Read the model definition and answer for the solid it produces. Units are mm, in the model's axes. Give positions to 0.01 mm unless a question says otherwise; leave off trailing zeros. Write each loop counter-clockwise with the first axis right and the second up, starting at its lowest first coordinate (ties: lowest second). Pieces come first, ordered by that corner, then holes. Notation, with made-up numbers: M 84.25,26.5 L 111.25,26.5 A6 cw 111.25,33.5 Z; hole C -11,8 d1. An arc over 180 degrees is marked long. Use a Markdown table: item, result. Add a question column.
Item 1: Consider probe 1 along Z at (x, y) = (10, 0.15); probe 2 along Z at (x, y) = (2, 0); probe 3 along X at (y, z) = (-0.15, -32). Determine where each line is inside the solid, lowest interval first. Write a range as [from, to].
Item 2: A cutting plane is placed at A-A on y = 0. Determine the outline of the cut face in (x, z).
Item 3: Given P1, Ø2.5, axis at x = -10.46, z = -5.9, coming from the +Y side, flat-ended and moving along its own axis, determine where the tip first touches the part or whether it passes through.
Item 4: A cutting plane is placed at B-B on z = -21.5. Determine the outline of the cut face in (x, y).
Item 5: The mould has two halves that part along X. Classify faces 1 (the cylindrical face through (-10.392, -0.004, -7.396)), 2 (the flat face through (9, 0, -22)), 3 (the cylindrical face through (0.062, 0.004, -35.055)), 4 (the flat face through (-9, 0, -22)): pulls with the +X half, pulls with the -X half, needs draft (parallel to the pull), parting line crosses it, or undercut.
Item 6: A cutting plane is placed at C-C on x = -4. Determine the outline of the cut face in (y, z).
from build123d import *

# Parameters (mm, degrees)
SKETCH1_R           = 1.5
BOSS_EXTRUDE1_DEPTH = 0.25


with BuildPart() as part:
    # Sketch1 → Boss-Extrude1 (new, symmetric)
    with BuildSketch(Plane(origin=(0, 0, 0), x_dir=(1, 0, 0), z_dir=(0, 1, 0))):
        with BuildLine():
            Line((0, 0), (7.05572809, 0))
            ThreePointArc((7.05572809, 0), (13.860934557, 3.794151103), (14.211145618, 11.577708764))
            Line((14.211145618, 11.577708764), (3.577708764, 32.844582472))
            ThreePointArc((3.577708764, 32.844582472), (0, 35.05572809), (-3.577708764, 32.844582472))
            Line((-3.577708764, 32.844582472), (-14.211145618, 11.577708764))
            ThreePointArc((-14.211145618, 11.577708764), (-13.860934557, 3.794151103), (-7.05572809, 0))
            Line((-7.05572809, 0), (0, 0))
        make_face()
        with Locations(Location((-10.458331323, 5.897075552, 0), (0, 0, 270))):
            Circle(SKETCH1_R, mode=Mode.SUBTRACT)
    extrude(amount=BOSS_EXTRUDE1_DEPTH, both=True)


solid = part.part
Filled in:
| question | item | result |
|---|---|---|
| 1 | probe 1 | [-20, -0.56] |
| 1 | probe 2 | [-34.52, 0] |
| 1 | probe 3 | [-4, 4] |
| 2 | outline | M -14.21,-11.58 L -3.58,-32.84 A4 ccw 3.58,-32.84 L 14.21,-11.58 A8 ccw 7.06,0 L -7.06,0 A8 ccw Z; hole C -10.46,-5.9 d3 |
| 3 | P1 | through |
| 4 | outline | M -9.25,-0.25 L 9.25,-0.25 L 9.25,0.25 L -9.25,0.25 Z |
| 5 | face 1 | undercut |
| 5 | face 2 | pulls with the +X half |
| 5 | face 3 | parting line crosses it |
| 5 | face 4 | pulls with the -X half |
| 6 | outline | M -0.25,-32 L 0.25,-32 L 0.25,0 L -0.25,0 Z |
